The model under review builds one solid part; all positions refer to its coordinate system, in mm. Face numbers are marked on the shaded views. A direction names the side the tool comes from. Round coordinates to 2 decimals unless told otherwise and drop trailing zeros. Write each loop counter-clockwise with the first axis right and the second up, starting at its lowest first coordinate (ties: lowest second). Pieces come first, ordered by that corner, then holes. Notation, with made-up numbers: (-27, -36.5) - (-8, -36.5) arc R11 ccw to (-8, -32.5) - close; hole circle Ø9 at (76, 54). An arc over 180 degrees is marked (long way). Write each question's results on one line, items separated by ' | '.
```python
from build123d import *

# Parameters (mm, degrees)
CUT_EXTRUDE1_REACH     = 213.303
SKETCH2_R              = 11.5
M24_TAPPED_HOLE1_D     = 21
M24_TAPPED_HOLE1_DEPTH = 17.6909635
M24_TAPPED_HOLE1_TIP   = 6.3090365
M12_TAPPED_HOLE1_D     = 10.2
M12_TAPPED_HOLE1_DEPTH = 8.935610843
M12_TAPPED_HOLE1_TIP   = 3.064389157


with BuildPart() as part:
    # Sketch1 → Revolve1 (revolve)
    with BuildSketch(Plane.XY, mode=Mode.PRIVATE) as revolve1_sk:
        Polygon((14, -37.771370899), (14, -8.704913174), (28, -0.622009405), (28, 49.228629101), (88, 49.228629101), (91.464101615, 43.228629101), (138, 43.228629101), (138, 15.228629101), (59.901806028, 15.228629101), (59.901806028, 9.228629101), (35, -37.771370899), align=None)
    revolve(revolve1_sk.sketch.rotate(Axis((0, 62.992349216, 0), (0, -1, 0)), 90), axis=Axis((0, 62.992349216, 0), (0, -1, 0)))

    # Sketch2 → Cut-Extrude1 (cut, up to next)
    with BuildSketch(Plane(origin=(0, 43.228629101, 0), x_dir=(1, 0, 0), z_dir=(0, 1, 0)), mode=Mode.PRIVATE) as cut_extrude1_sk1:
        with Locations(Location((0, 112.5, 0), (0, 0, 270))):
            Circle(SKETCH2_R)
    cut_extrude1_tool1 = extrude(cut_extrude1_sk1.sketch, amount=-CUT_EXTRUDE1_REACH, mode=Mode.PRIVATE) & part.part
    # Sketch2 → Cut-Extrude1 (cut, up to next)
    with BuildSketch(Plane(origin=(0, 43.228629101, 0), x_dir=(1, 0, 0), z_dir=(0, 1, 0)), mode=Mode.PRIVATE) as cut_extrude1_sk2:
        with Locations(Location((97.427857926, 56.25, 0), (0, 0, 270))):
            Circle(SKETCH2_R)
    cut_extrude1_tool2 = extrude(cut_extrude1_sk2.sketch, amount=-CUT_EXTRUDE1_REACH, mode=Mode.PRIVATE) & part.part
    # Sketch2 → Cut-Extrude1 (cut, up to next)
    with BuildSketch(Plane(origin=(0, 43.228629101, 0), x_dir=(1, 0, 0), z_dir=(0, 1, 0)), mode=Mode.PRIVATE) as cut_extrude1_sk3:
        with Locations(Location((97.427857926, -56.25, 0), (0, 0, 270))):
            Circle(SKETCH2_R)
    cut_extrude1_tool3 = extrude(cut_extrude1_sk3.sketch, amount=-CUT_EXTRUDE1_REACH, mode=Mode.PRIVATE) & part.part
    # Sketch2 → Cut-Extrude1 (cut, up to next)
    with BuildSketch(Plane(origin=(0, 43.228629101, 0), x_dir=(1, 0, 0), z_dir=(0, 1, 0)), mode=Mode.PRIVATE) as cut_extrude1_sk4:
        with Locations(Location((0, -112.5, 0), (0, 0, 270))):
            Circle(SKETCH2_R)
    cut_extrude1_tool4 = extrude(cut_extrude1_sk4.sketch, amount=-CUT_EXTRUDE1_REACH, mode=Mode.PRIVATE) & part.part
    # Sketch2 → Cut-Extrude1 (cut, up to next)
    with BuildSketch(Plane(origin=(0, 43.228629101, 0), x_dir=(1, 0, 0), z_dir=(0, 1, 0)), mode=Mode.PRIVATE) as cut_extrude1_sk5:
        with Locations(Location((-97.427857926, -56.25, 0), (0, 0, 270))):
            Circle(SKETCH2_R)
    cut_extrude1_tool5 = extrude(cut_extrude1_sk5.sketch, amount=-CUT_EXTRUDE1_REACH, mode=Mode.PRIVATE) & part.part
    # Sketch2 → Cut-Extrude1 (cut, up to next)
    with BuildSketch(Plane(origin=(0, 43.228629101, 0), x_dir=(1, 0, 0), z_dir=(0, 1, 0)), mode=Mode.PRIVATE) as cut_extrude1_sk6:
        with Locations(Location((-97.427857926, 56.25, 0), (0, 0, 270))):
            Circle(SKETCH2_R)
    cut_extrude1_tool6 = extrude(cut_extrude1_sk6.sketch, amount=-CUT_EXTRUDE1_REACH, mode=Mode.PRIVATE) & part.part
    add(cut_extrude1_tool1.solids().sort_by_distance((0, 43.228629, -112.5))[0], mode=Mode.SUBTRACT)
    add(cut_extrude1_tool2.solids().sort_by_distance((97.427858, 43.228629, -56.25))[0], mode=Mode.SUBTRACT)
    add(cut_extrude1_tool3.solids().sort_by_distance((97.427858, 43.228629, 56.25))[0], mode=Mode.SUBTRACT)
    add(cut_extrude1_tool4.solids().sort_by_distance((0, 43.228629, 112.5))[0], mode=Mode.SUBTRACT)
    add(cut_extrude1_tool5.solids().sort_by_distance((-97.427858, 43.228629, 56.25))[0], mode=Mode.SUBTRACT)
    add(cut_extrude1_tool6.solids().sort_by_distance((-97.427858, 43.228629, -56.25))[0], mode=Mode.SUBTRACT)

    # M24 Tapped Hole1
    with Locations(Plane(origin=(0, 49.228629101, -60), x_dir=(0, 0, 1), z_dir=(0, 1, 0))):
        with Locations((0, 0), (120, 0)):
            Hole(M24_TAPPED_HOLE1_D / 2, depth=M24_TAPPED_HOLE1_DEPTH)
            with Locations((0, 0, -(M24_TAPPED_HOLE1_DEPTH + M24_TAPPED_HOLE1_TIP / 2))):  # 118° drill point
                Cone(0, M24_TAPPED_HOLE1_D / 2, M24_TAPPED_HOLE1_TIP, mode=Mode.SUBTRACT)

    # M12 Tapped Hole1
    with Locations(Plane(origin=(-44, 49.228629101, 0), x_dir=(0, 0, 1), z_dir=(0, 1, 0))):
        with Locations((0, 0), (0, 88)):
            Hole(M12_TAPPED_HOLE1_D / 2, depth=M12_TAPPED_HOLE1_DEPTH)
            with Locations((0, 0, -(M12_TAPPED_HOLE1_DEPTH + M12_TAPPED_HOLE1_TIP / 2))):  # 118° drill point
                Cone(0, M12_TAPPED_HOLE1_D / 2, M12_TAPPED_HOLE1_TIP, mode=Mode.SUBTRACT)


solid = part.part
```
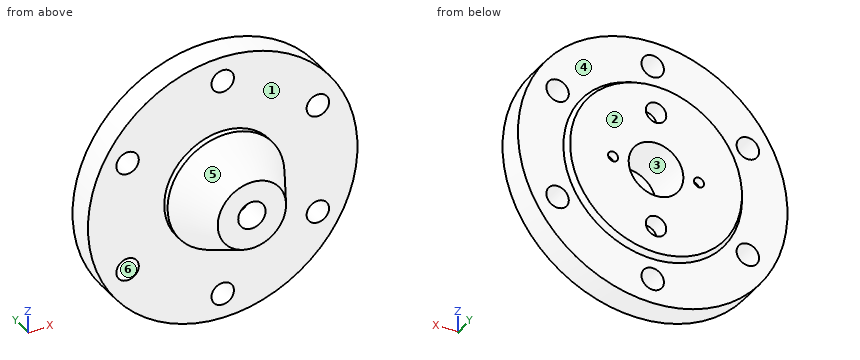
Q1. Insertion check: P1, Ø10, axis at x = 97, y = 36.5, coming from the -Z side; P2, Ø6, axis at x = 44, z = 0, coming from the +Y side; P3, Ø25, axis at x = 0, z = 0, coming from the -Y side; P4, Ø4, axis at x = -27, z = -92, coming from the +Y side. Each pin has a flat end and moves straight along its axis. Give the tip position at first contact, or say it passes through.
Evaluation:
P1: stops at z = -102.86 | P2: stops at y = 39.03 | P3: passes through | P4: stops at y = 43.23
Q2. We need section C-C (z = -56.25). State how many separate pieces and enclosed holes the cut face has, plus the area to 3 significant figures.
Evaluation:
separate pieces: 3 | enclosed holes: 0 | area: 6,650 mm^2
Q3. We need section A-A (z = -112.5). State the section outline as (x, y) points, plus the area to 3 significant figures.
Evaluation:
outline: (-79.92, 15.23) - (-11.5, 15.23) - (-11.5, 43.23) - (-79.92, 43.23) - close; (11.5, 15.23) - (79.92, 15.23) - (79.92, 43.23) - (11.5, 43.23) - close | area: 3,830 mm^2
Q4. The part is to be moulded in two halves that separate along X. For the marked faces 4, 5 and 6, say which applies: released by +X, released by -X, zero draft, split by the parting line, or undercut.
Evaluation:
face 4: zero draft | face 5: split by the parting line | face 6: undercut
Q5. Tool access review of the marked faces 1, 2 and 3: name each direction out of +Z, -Z, +X, -X, +Y, -Y from which nothing blocks a thin tool from reaching the whole face with its end or side.
Evaluation:
face 1: -Y | face 2: +Z, -Z, +X, -X, +Y | face 3: +Y
Q6. For probe 1 along X at (y, z) = (35.5, 60); probe 2 along X at (y, z) = (47, 0); probe 3 along X at (y, z) = (25.5, 56.25), list the stretches that pass through material, from the lowest coordinate up.
Evaluation:
probe 1: x = -124.27 to -108.3, -86.56 to -10.5, 10.5 to 86.56, 108.3 to 124.27 | probe 2: x = -89.29 to -49.1, -38.9 to -28, 28 to 38.9, 49.1 to 89.29 | probe 3: x = -126.02 to -108.93, -85.93 to 85.93, 108.93 to 126.02
Q7. We need section B-B (y = -23). State the section outline as (x, z) points.
Evaluation:
outline: circle Ø85.65 at (0, 0); hole circle Ø28 at (0, 0)
